Check sheet for the drawn part. Datum: minimum x, y, z corner. Units: mm. A direction names the side the tool comes from. Coordinates: 2 decimals unless noted, no trailing zeros. Order: outer loops, then holes, each group sorted by start corner. A loop starts at its lowest first (then second) coordinate and runs counter-clockwise, first axis right, second up. Notation, with made-up numbers: (-31.5, 46) - (1.5, 46) arc R29 ccw to (1.5, 73) - close; hole circle Ø1 at (78, -26). An arc over 180 degrees is marked (long way). Put each result on its own line as item: value.
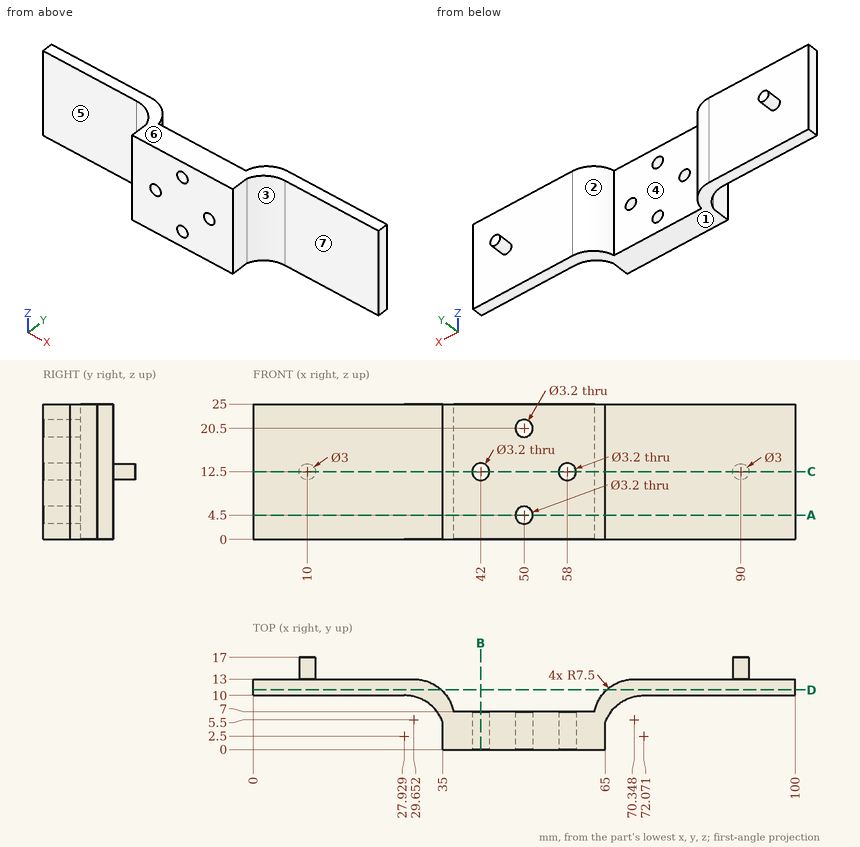
Q1. Thickness scan on L1, parallel to X at y = 2.5, z = 12.5; L2, parallel to X at y = 2.75, z = 20.5; L3, parallel to X at y = 5.25, z = 13 (1 decimal). Record the ranges inside material, lowest first. Write a range as [from, to].
Answer block:
L1: x = [35, 40.4], [43.6, 56.4], [59.6, 65]
L2: x = [35, 48.4], [51.6, 65]
L3: x = [34.9, 40.5], [43.5, 56.5], [59.5, 65.1]
Q2. Depth check by flat-ended pin: pin 1 Ø5 at (x, z) = (62, 9) entering from +Y (1 decimal); pin 2 Ø8 at (y, z) = (3, 20) entering from +X; pin 3 Ø4 at (x, y) = (45, 9.5) entering from -Z; pin 4 Ø2.5 at (y, z) = (3, 10.5) entering from -X. Enter the tip coordinate at first touch or a pass-through.
Answer block:
pin 1: stops at y = 10.2
pin 2: stops at x = 66.07
pin 3: passes through
pin 4: stops at x = 35
Q3. Section check D-D on y = 11. Record the boundary of the cut face in (x, z).
Answer block:
outline: (0, 0) - (34.75, 0) - (34.75, 25) - (0, 25) - close; (65.25, 0) - (100, 0) - (100, 25) - (65.25, 25) - close
Q4. Section check A-A on z = 4.5. Record the boundary of the cut face in (x, y).
Answer block:
outline: (0, 10) - (27.93, 10) arc R7.5 cw to (35, 5) - (35, 0) - (48.4, 0) - (48.4, 7) - (37, 7) arc R7.5 ccw to (29.65, 13) - (0, 13) - close; (51.6, 0) - (65, 0) - (65, 5) arc R7.5 cw to (72.07, 10) - (100, 10) - (100, 13) - (70.35, 13) arc R7.5 ccw to (63, 7) - (51.6, 7) - close
Q5. Section check C-C on z = 12.5. State how many separate pieces and enclosed holes the cut face has, then the cut area to 3 significant figures.
Answer block:
separate pieces: 3
enclosed holes: 0
area: 420 mm^2
Q6. Section check B-B on x = 42. Record the boundary of the cut face in (y, z).
Answer block:
outline: (0, 0) - (7, 0) - (7, 10.9) - (0, 10.9) - close; (0, 14.1) - (7, 14.1) - (7, 25) - (0, 25) - close
Q7. Draft check along X on the marked faces 1, 2 and 3. Enter one of: pulls with the +X half, pulls with the -X half, needs draft (parallel to the pull), parting line crosses it, or undercut.
Answer block:
face 1: needs draft
face 2: undercut
face 3: pulls with the +X half
Q8. Access from +Z, -Z, +X, -X, +Y, -Y to the whole of each face (thin tool, end or side, straight path). Record for the marked faces 4, 5, 6 and 7.
Answer block:
face 4: +Z, -Z, +Y
face 5: +Z, -Z, -X, -Y
face 6: +Z, +X, -X, +Y, -Y
face 7: +Z, -Z, +X, -Y
